Autodesk Inventor part; units mm, degrees
ref_plane "YZ Plane" through (0, 0, 0) normal (1, 0, 0) x (0, 1, 0)
ref_plane "XZ Plane" through (0, 0, 0) normal (0, 1, 0) x (-1, 0, 0)
ref_plane "XY Plane" through (0, 0, 0) normal (0, 0, 1) x (1, 0, 0)
sketch "Sketch1" plane through (0, 0, 0) normal (0, 0, 1) x (1, 0, 0)
  line L0 (-28.4765, -2.55) -> (28.4765, -2.55)
  arc A0 (44.7, -18.7735) -> (28.4765, -2.55) centre (0, -47.25) ccw
  line L1 (44.7, -18.7735) -> (44.7, -75.7265)
  arc A1 (28.4765, -91.95) -> (44.7, -75.7265) centre (0, -47.25) ccw
  line L2 (28.4765, -91.95) -> (-28.4765, -91.95)
  arc A2 (-44.7, -75.7265) -> (-28.4765, -91.95) centre (0, -47.25) ccw
  line L3 (-44.7, -75.7265) -> (-44.7, -18.7735)
  arc A3 (-28.4765, -2.55) -> (-44.7, -18.7735) centre (0, -47.25) ccw
  line L4 (-28.4765, 91.95) -> (28.4765, 91.95)
  arc A4 (44.7, 75.7265) -> (28.4765, 91.95) centre (0, 47.25) ccw
  line L5 (44.7, 75.7265) -> (44.7, 18.7735)
  arc A5 (28.4765, 2.55) -> (44.7, 18.7735) centre (0, 47.25) ccw
  line L6 (28.4765, 2.55) -> (-28.4765, 2.55)
  arc A6 (-44.7, 18.7735) -> (-28.4765, 2.55) centre (0, 47.25) ccw
  line L7 (-44.7, 18.7735) -> (-44.7, 75.7265)
  arc A7 (-28.4765, 91.95) -> (-44.7, 75.7265) centre (0, 47.25) ccw
  line L8 (-28.4765, 186.45) -> (28.4765, 186.45)
  arc A8 (44.7, 170.2265) -> (28.4765, 186.45) centre (0, 141.75) ccw
  line L9 (44.7, 170.2265) -> (44.7, 113.2735)
  arc A9 (28.4765, 97.05) -> (44.7, 113.2735) centre (0, 141.75) ccw
  line L10 (28.4765, 97.05) -> (-28.4765, 97.05)
  arc A10 (-44.7, 113.2735) -> (-28.4765, 97.05) centre (0, 141.75) ccw
  line L11 (-44.7, 113.2735) -> (-44.7, 170.2265)
  arc A11 (-28.4765, 186.45) -> (-44.7, 170.2265) centre (0, 141.75) ccw
  circle A12 centre (-41.25, -88.5) radius 2.25
  circle A13 centre (41.25, -88.5) radius 2.25
  circle A14 centre (41.25, -6) radius 2.25
  circle A15 centre (-41.25, -6) radius 2.25
  circle A16 centre (-41.25, 6) radius 2.25
  circle A17 centre (41.25, 6) radius 2.25
  circle A18 centre (41.25, 88.5) radius 2.25
  circle A19 centre (-41.25, 88.5) radius 2.25
  circle A20 centre (41.25, 183) radius 2.25
  circle A21 centre (41.25, 100.5) radius 2.25
  circle A22 centre (-41.25, 100.5) radius 2.25
  circle A23 centre (-41.25, 183) radius 2.25
  arc A24 (15.0245, 209.46) -> (15.0245, 194.54) centre (17.5, 202) ccw
  line L12 (15.0245, 209.46) -> (19.9755, 209.46)
  arc A25 (19.9755, 194.54) -> (19.9755, 209.46) centre (17.5, 202) ccw
  line L13 (19.9755, 194.54) -> (15.0245, 194.54)
  arc A26 (-15.0245, 194.54) -> (-15.0245, 209.46) centre (-17.5, 202) ccw
  line L14 (-15.0245, 194.54) -> (-19.9755, 194.54)
  arc A27 (-19.9755, 209.46) -> (-19.9755, 194.54) centre (-17.5, 202) ccw
  line L15 (-19.9755, 209.46) -> (-15.0245, 209.46)
  line L16 (-54.7, 214.7) -> (54.7, 214.7)
  line L17 (54.7, -129.8) -> (-54.7, -129.8)
  line L18 (-78, -129.8) -> (78, -129.8)
  line L19 (-78, -129.8) -> (-78, 214.7)
  arc A28 (-64.7298, -120.3577) -> (-68.5577, -116.5298) centre (-66.3, -118.1) ccw
  arc A29 (-70.1472, -118.8153) -> (-67.0153, -121.9472) centre (-68.3, -120.1) ccw
  line L20 (-67.0153, -121.9472) -> (-64.7298, -120.3577)
  line L21 (-70.1472, -118.8153) -> (-68.5577, -116.5298)
  arc A30 (68.5577, -116.5298) -> (64.7298, -120.3577) centre (66.3, -118.1) ccw
  arc A31 (67.0153, -121.9472) -> (70.1472, -118.8153) centre (68.3, -120.1) ccw
  line L22 (67.0153, -121.9472) -> (64.7298, -120.3577)
  line L23 (70.1472, -118.8153) -> (68.5577, -116.5298)
  line L24 (78, -129.8) -> (78, 214.7)
  arc A32 (-68.5577, 201.4298) -> (-64.7298, 205.2577) centre (-66.3, 203) ccw
  arc A33 (-67.0153, 206.8472) -> (-70.1472, 203.7153) centre (-68.3, 205) ccw
  line L25 (-67.0153, 206.8472) -> (-64.7298, 205.2577)
  line L26 (-70.1472, 203.7153) -> (-68.5577, 201.4298)
  line L27 (70.1472, 203.7153) -> (68.5577, 201.4298)
  arc A34 (64.7298, 205.2577) -> (68.5577, 201.4298) centre (66.3, 203) ccw
  line L28 (67.0153, 206.8472) -> (64.7298, 205.2577)
  arc A35 (70.1472, 203.7153) -> (67.0153, 206.8472) centre (68.3, 205) ccw
  line L29 (-78, 214.7) -> (78, 214.7)
  point P0 (-54.7, -129.8)
  point P1 (54.7, -129.8)
  point P2 (0, 205.2577)
  dimension "d197" = 156
  dimension "d199" = 344.5
  dimension "d221" = 344.5
  dimension "d224" = 9.7
  dimension "d225" = 9.7
  dimension "d228" = 11.7
  dimension "d229" = 11.7
  dimension "d232" = 5.5
  dimension "d233" = 4.5
extrude "Extrusion1" add sketch "Sketch1" along normal blind 3
sketch "Sketch2" plane through (0, 0, 3) normal (0, 0, 1) x (1, 0, 0)
  line L0 (28.4765, 97.05) -> (-28.4765, 97.05)
  arc A0 (-44.7, 113.2735) -> (-28.4765, 97.05) centre (0, 141.75) ccw
  line L1 (-44.7, 113.2735) -> (-44.7, 170.2265)
  arc A1 (-28.4765, 186.45) -> (-44.7, 170.2265) centre (0, 141.75) ccw
  line L2 (-28.4765, 186.45) -> (28.4765, 186.45)
  arc A2 (44.7, 170.2265) -> (28.4765, 186.45) centre (0, 141.75) ccw
  line L3 (44.7, 170.2265) -> (44.7, 113.2735)
  arc A3 (28.4765, 97.05) -> (44.7, 113.2735) centre (0, 141.75) ccw
  line L4 (44.7, 75.7265) -> (44.7, 18.7735)
  arc A4 (28.4765, 2.55) -> (44.7, 18.7735) centre (0, 47.25) ccw
  line L5 (28.4765, 2.55) -> (-28.4765, 2.55)
  arc A5 (-44.7, 18.7735) -> (-28.4765, 2.55) centre (0, 47.25) ccw
  line L6 (-44.7, 18.7735) -> (-44.7, 75.7265)
  arc A6 (-28.4765, 91.95) -> (-44.7, 75.7265) centre (0, 47.25) ccw
  line L7 (-28.4765, 91.95) -> (28.4765, 91.95)
  arc A7 (44.7, 75.7265) -> (28.4765, 91.95) centre (0, 47.25) ccw
  arc A8 (28.4765, -91.95) -> (44.7, -75.7265) centre (0, -47.25) ccw
  line L8 (28.4765, -91.95) -> (-28.4765, -91.95)
  arc A9 (-44.7, -75.7265) -> (-28.4765, -91.95) centre (0, -47.25) ccw
  line L9 (-44.7, -75.7265) -> (-44.7, -18.7735)
  arc A10 (-28.4765, -2.55) -> (-44.7, -18.7735) centre (0, -47.25) ccw
  line L10 (-28.4765, -2.55) -> (28.4765, -2.55)
  arc A11 (44.7, -18.7735) -> (28.4765, -2.55) centre (0, -47.25) ccw
  line L11 (44.7, -18.7735) -> (44.7, -75.7265)
  line L12 (-15.0245, 194.54) -> (-19.9755, 194.54)
  arc A12 (-19.9755, 209.46) -> (-19.9755, 194.54) centre (-17.5, 202) ccw
  line L13 (-19.9755, 209.46) -> (-15.0245, 209.46)
  arc A13 (-15.0245, 194.54) -> (-15.0245, 209.46) centre (-17.5, 202) ccw
  line L14 (15.0245, 209.46) -> (19.9755, 209.46)
  arc A14 (19.9755, 194.54) -> (19.9755, 209.46) centre (17.5, 202) ccw
  line L15 (19.9755, 194.54) -> (15.0245, 194.54)
  arc A15 (15.0245, 209.46) -> (15.0245, 194.54) centre (17.5, 202) ccw
  arc A16 (64.7298, 205.2577) -> (68.5577, 201.4298) centre (66.3, 203) ccw
  line L16 (64.7298, 205.2577) -> (67.0153, 206.8472)
  arc A17 (70.1472, 203.7153) -> (67.0153, 206.8472) centre (68.3, 205) ccw
  line L17 (70.1472, 203.7153) -> (68.5577, 201.4298)
  arc A18 (-67.0153, 206.8472) -> (-70.1472, 203.7153) centre (-68.3, 205) ccw
  line L18 (-67.0153, 206.8472) -> (-64.7298, 205.2577)
  arc A19 (-68.5577, 201.4298) -> (-64.7298, 205.2577) centre (-66.3, 203) ccw
  line L19 (-68.5577, 201.4298) -> (-70.1472, 203.7153)
  arc A20 (67.0153, -121.9472) -> (70.1472, -118.8153) centre (68.3, -120.1) ccw
  line L20 (67.0153, -121.9472) -> (64.7298, -120.3577)
  arc A21 (68.5577, -116.5298) -> (64.7298, -120.3577) centre (66.3, -118.1) ccw
  line L21 (68.5577, -116.5298) -> (70.1472, -118.8153)
  arc A22 (-64.7298, -120.3577) -> (-68.5577, -116.5298) centre (-66.3, -118.1) ccw
  line L22 (-64.7298, -120.3577) -> (-67.0153, -121.9472)
  arc A23 (-70.1472, -118.8153) -> (-67.0153, -121.9472) centre (-68.3, -120.1) ccw
  line L23 (-70.1472, -118.8153) -> (-68.5577, -116.5298)
  circle A24 centre (41.25, 6) radius 2.25
  circle A25 centre (41.25, 100.5) radius 2.25
  circle A26 centre (41.25, 88.5) radius 2.25
  circle A27 centre (-41.25, 100.5) radius 2.25
  circle A28 centre (-41.25, 88.5) radius 2.25
  circle A29 centre (-41.25, 6) radius 2.25
  circle A30 centre (-41.25, -6) radius 2.25
  circle A31 centre (41.25, -6) radius 2.25
  circle A32 centre (41.25, 183) radius 2.25
  circle A33 centre (-41.25, 183) radius 2.25
  circle A34 centre (41.25, -88.5) radius 2.25
  circle A35 centre (-41.25, -88.5) radius 2.25
  line L24 (-78, -129.8) -> (78, -129.8)
  line L25 (78, -129.8) -> (78, 214.7)
  line L26 (78, 214.7) -> (-78, 214.7)
  line L27 (-78, 214.7) -> (-78, -129.8)
  point P0 (0, 0)
extrude "Extrusion2" add sketch "Sketch2" against normal up to surface (3 mm away) contours L12 A12 L13 A13 | L14 A14 L15 A15
equation "\"d221\" = d199"
properties part number "front_panel2"
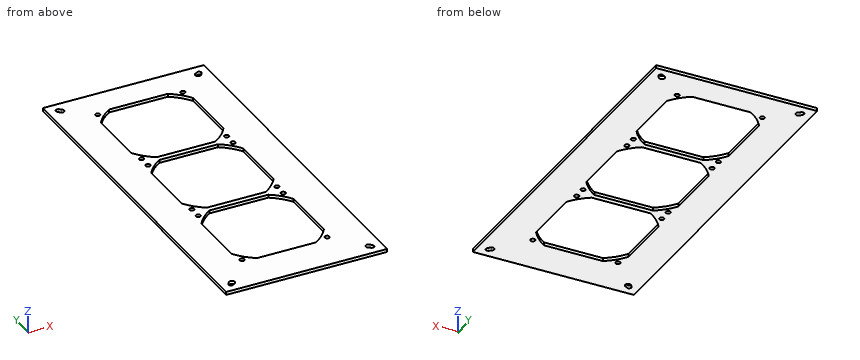
The listing builds one solid part. Answer for the finished solid, in the listing's coordinates (mm). Coordinates: 2 decimals unless noted, no trailing zeros. Write each loop counter-clockwise with the first axis right and the second up, starting at its lowest first coordinate (ties: lowest second). Pieces come first, ordered by that corner, then holes. Notation, with made-up numbers: (62.25, 15.25) - (73.25, 15.25) arc R14 cw to (73.25, 23.25) - close; hole circle Ø1 at (80, 50.25). An arc over 180 degrees is marked (long way). Put each result on its own line as item: value.
1. The part is cut by section D-D on x = 32.5. Give the vertices of the cut face in (y, z).
Answer sheet:
outline: (-129.8, 0) - (-89.12, 0) - (-89.12, 3) - (-129.8, 3) - close; (-5.38, 0) - (5.38, 0) - (5.38, 3) - (-5.38, 3) - close; (89.12, 0) - (99.88, 0) - (99.88, 3) - (89.12, 3) - close; (183.62, 0) - (214.7, 0) - (214.7, 3) - (183.62, 3) - close
2. The part is cut by section B-B on y = 155.5. Give the vertices of the cut face in (x, z).
Answer sheet:
outline: (-78, 0) - (-44.7, 0) - (-44.7, 3) - (-78, 3) - close; (44.7, 0) - (78, 0) - (78, 3) - (44.7, 3) - close
3. The part is cut by section C-C on z = 1.4. State how many separate pieces and enclosed holes the cut face has, plus the area to 3 significant figures.
Answer sheet:
separate pieces: 1
enclosed holes: 19
area: 30,800 mm^2
4. The part is cut by section A-A on x = -16.5. Give the vertices of the cut face in (y, z), plus the area to 3 significant figures.
Answer sheet:
outline: (-129.8, 0) - (-91.95, 0) - (-91.95, 3) - (-129.8, 3) - close; (-2.55, 0) - (2.55, 0) - (2.55, 3) - (-2.55, 3) - close; (91.95, 0) - (97.05, 0) - (97.05, 3) - (91.95, 3) - close; (186.45, 0) - (214.7, 0) - (214.7, 3) - (186.45, 3) - close
area: 229 mm^2
5. Find the intervals of material crossed by line 1 along Y through (x, z) = (-22, 1); line 2 along X through (y, z) = (-37, 0.4); line 3 along X through (y, z) = (182.5, 1.95), in increasing order. Write a range as from..to.
Answer sheet:
line 1: y = -129.8..-91.95, -2.55..2.55, 91.95..97.05, 186.45..214.7
line 2: x = -78..-44.7, 44.7..78
line 3: x = -78..-43.44, -39.06..-33.89, 33.89..39.06, 43.44..78
6. A flat-ended cylindrical pin translates along its axis: pin 1 Ø4.5 at (x, y) = (-66.3, 203) entering from +Z. Find the tip coordinate at first contact, or state that the pin passes through.
Answer sheet:
pin 1: passes through
